Geometry: final body of the model. Coordinates: model frame, mm. Give positions to 0.01 mm unless a question says otherwise; leave off trailing zeros. Loops run counter-clockwise (first coordinate to the right, second up) from the corner with the lowest first, then second, coordinate; pieces in that order, holes last. Notation, with made-up numbers: (51, -11) -> (97, -11) arc R9 ccw to (97, 2) -> close; hole circle Ø11 at (2.5, 82.5). An arc over 180 degrees is marked (long way). Answer in a Markdown table with one row per item. Add a question column.
1) Section query B-B (x = 1135). Return the cut outline in (y, z).
2) Section query A-A (y = -343.5). Return the cut outline in (x, z), plus the area to 3 significant figures.
3) Section query C-C (z = 12). Return the cut outline in (x, y).
4) Line query: line 1 (X direction, y = -391.5, z = 23); line 2 (X direction, y = -536.5, z = 10.5); line 3 (Y direction, x = 955, z = 12.5). Output: solid intervals per line, ascending. Write a range as from..to.
```python
from build123d import *

# Parameters (mm, degrees)
F0_W     = 620
F0_H     = 40
F1_DEPTH = 1800
F3_DEPTH = 40.001


# Not quite as in the source:
# - a feature of the source that left no trace in its solid (it failed there, or was rolled back) is left out


with BuildPart() as f1:
    # F0 (on Right) → F1 (new body)
    with BuildSketch(Plane.YZ):
        with Locations((-310, 20)):
            Rectangle(F0_W, F0_H)
    extrude(amount=F1_DEPTH)

    # F2 (on face) → F3 (cut, through all)
    with BuildSketch(Plane.XY.offset(40)):
        with BuildLine():
            Line((960, -100), (640, -100))
            ThreePointArc((640, -100), (629.3933982822, -104.3933982822), (625, -115))
            Line((625, -115), (625, -535))
            ThreePointArc((625, -535), (629.3933982822, -545.6066017178), (640, -550))
            Line((640, -550), (960, -550))
            ThreePointArc((960, -550), (970.6066017178, -545.6066017178), (975, -535))
            Line((975, -535), (975, -115))
            ThreePointArc((975, -115), (970.6066017178, -104.3933982822), (960, -100))
        make_face()
        with BuildLine():
            Line((1160, -100), (1040, -100))
            ThreePointArc((1040, -100), (1029.3933982822, -104.3933982822), (1025, -115))
            Line((1025, -115), (1025, -535))
            ThreePointArc((1025, -535), (1029.3933982822, -545.6066017178), (1040, -550))
            Line((1040, -550), (1160, -550))
            ThreePointArc((1160, -550), (1170.6066017178, -545.6066017178), (1175, -535))
            Line((1175, -535), (1175, -115))
            ThreePointArc((1175, -115), (1170.6066017178, -104.3933982822), (1160, -100))
        make_face()
    extrude(amount=-F3_DEPTH, mode=Mode.SUBTRACT)


solid = f1.part
```
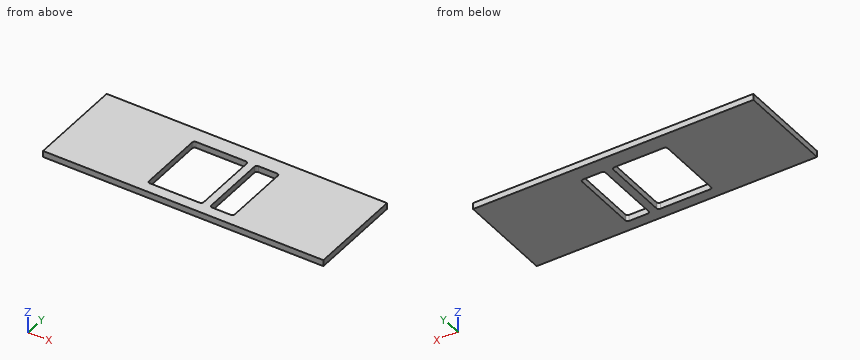
Evaluation:
| question | item | result |
|---|---|---|
| 1 | outline | (-620, 0) -> (-550, 0) -> (-550, 40) -> (-620, 40) -> close; (-100, 0) -> (0, 0) -> (0, 40) -> (-100, 40) -> close |
| 2 | outline | (0, 0) -> (625, 0) -> (625, 40) -> (0, 40) -> close; (975, 0) -> (1025, 0) -> (1025, 40) -> (975, 40) -> close; (1175, 0) -> (1800, 0) -> (1800, 40) -> (1175, 40) -> close |
| 2 | area | 52,000 mm² |
| 3 | outline | (0, -620) -> (1800, -620) -> (1800, 0) -> (0, 0) -> close; hole (625, -535) arc R15 ccw to (640, -550) -> (960, -550) arc R15 ccw to (975, -535) -> (975, -115) arc R15 ccw to (960, -100) -> (640, -100) arc R15 ccw to (625, -115) -> close; hole (1025, -535) arc R15 ccw to (1040, -550) -> (1160, -550) arc R15 ccw to (1175, -535) -> (1175, -115) arc R15 ccw to (1160, -100) -> (1040, -100) arc R15 ccw to (1025, -115) -> close |
| 4 | line 1 | 0..625, 975..1025, 1175..1800 |
| 4 | line 2 | 0..625.08, 974.92..1025.08, 1174.92..1800 |
| 4 | line 3 | -620..-550, -100..0 |
